Could you check a few things on this model? Use its own coordinates, in mm. Coordinates: 2 decimals unless noted, no trailing zeros. Loops run counter-clockwise (first coordinate to the right, second up) from the corner with the lowest first, then second, coordinate; pieces in that order, holes last. Notation, with made-up numbers: (60, 53) - (64, 53) arc R13 ccw to (64, 62) - close; hole circle Ø3 at (79, -2). An arc over 180 degrees is marked (long way). One line per item, written item: value. Start each with the question number.
(1) If we section it at A-A on z = -7.5: Count the separate pieces of the cut face and the enclosed holes in it, then the cut area to 3 significant figures.
(2) If we section it at B-B on x = 55.5: Write out the boundary of the cut face in (y, z), then the cut area to 3 significant figures.
(3) If I drill on line 1 along Z through (x, y) = (117.5, -1); line 2 along Z through (x, y) = (74, 1.05), over which ranges is the centre line in solid material (lowest first)? Write a range as from..to.
(4) I'm going to push a flat-ended pin straight in: P1, Ø1.5, axis at x = 102.5, y = 0.5, coming from the +Z side. Where does the tip first touch, or does it pass through?
```python
from build123d import *

# Parameters (mm, degrees)
F1_W          = 145.2
F1_H          = 32
F2_DEPTH      = 2
F3_DEPTH      = 2.001
F3_DEPTH_BACK = 2.001
F4_R          = 1


with BuildPart() as f2:
    # F1 (on Front) → F2 (new body, symmetric)
    with BuildSketch(Plane.XZ):
        with Locations((67.15, -2.5)):
            Rectangle(F1_W, F1_H)
    extrude(amount=F2_DEPTH, both=True)

    # F0 (on Front) → F3 (cut, two sides)
    with BuildSketch(Plane.XZ) as f3_sk:
        with BuildLine():
            Line((2.45, -12.5), (2.45, 13.5))
            Line((2.45, 13.5), (-2.45, 13.5))
            Line((-2.45, 13.5), (-2.45, -12.5))
            ThreePointArc((-2.45, -12.5), (-2.1571067812, -13.2071067812), (-1.45, -13.5))
            Line((-1.45, -13.5), (1.45, -13.5))
            ThreePointArc((1.45, -13.5), (2.1571067812, -13.2071067812), (2.45, -12.5))
        make_face()
        with BuildLine():
            Line((10.35, 13.5), (5.45, 13.5))
            Line((5.45, 13.5), (5.45, -12.5))
            ThreePointArc((5.45, -12.5), (5.7428932188, -13.2071067812), (6.45, -13.5))
            Line((6.45, -13.5), (9.35, -13.5))
            ThreePointArc((9.35, -13.5), (10.0571067812, -13.2071067812), (10.35, -12.5))
            Line((10.35, -12.5), (10.35, 13.5))
        make_face()
        with BuildLine():
            Line((18.25, 13.5), (13.35, 13.5))
            Line((13.35, 13.5), (13.35, -12.5))
            ThreePointArc((13.35, -12.5), (13.6428932188, -13.2071067812), (14.35, -13.5))
            Line((14.35, -13.5), (17.25, -13.5))
            ThreePointArc((17.25, -13.5), (17.9571067812, -13.2071067812), (18.25, -12.5))
            Line((18.25, -12.5), (18.25, 13.5))
        make_face()
        with BuildLine():
            Line((26.15, 13.5), (21.25, 13.5))
            Line((21.25, 13.5), (21.25, -12.5))
            ThreePointArc((21.25, -12.5), (21.5428932188, -13.2071067812), (22.25, -13.5))
            Line((22.25, -13.5), (25.15, -13.5))
            ThreePointArc((25.15, -13.5), (25.8571067812, -13.2071067812), (26.15, -12.5))
            Line((26.15, -12.5), (26.15, 13.5))
        make_face()
        with BuildLine():
            Line((34.05, 13.5), (29.15, 13.5))
            Line((29.15, 13.5), (29.15, -12.5))
            ThreePointArc((29.15, -12.5), (29.4428932188, -13.2071067812), (30.15, -13.5))
            Line((30.15, -13.5), (33.05, -13.5))
            ThreePointArc((33.05, -13.5), (33.7571067812, -13.2071067812), (34.05, -12.5))
            Line((34.05, -12.5), (34.05, 13.5))
        make_face()
        with BuildLine():
            Line((41.95, 13.5), (37.05, 13.5))
            Line((37.05, 13.5), (37.05, -12.5))
            ThreePointArc((37.05, -12.5), (37.3428932188, -13.2071067812), (38.05, -13.5))
            Line((38.05, -13.5), (40.95, -13.5))
            ThreePointArc((40.95, -13.5), (41.6571067812, -13.2071067812), (41.95, -12.5))
            Line((41.95, -12.5), (41.95, 13.5))
        make_face()
        with BuildLine():
            Line((49.85, 13.5), (44.95, 13.5))
            Line((44.95, 13.5), (44.95, -12.5))
            ThreePointArc((44.95, -12.5), (45.2428932188, -13.2071067812), (45.95, -13.5))
            Line((45.95, -13.5), (48.85, -13.5))
            ThreePointArc((48.85, -13.5), (49.5571067812, -13.2071067812), (49.85, -12.5))
            Line((49.85, -12.5), (49.85, 13.5))
        make_face()
        with BuildLine():
            Line((57.75, 13.5), (52.85, 13.5))
            Line((52.85, 13.5), (52.85, -12.5))
            ThreePointArc((52.85, -12.5), (53.1428932188, -13.2071067812), (53.85, -13.5))
            Line((53.85, -13.5), (56.75, -13.5))
            ThreePointArc((56.75, -13.5), (57.4571067812, -13.2071067812), (57.75, -12.5))
            Line((57.75, -12.5), (57.75, 13.5))
        make_face()
        with BuildLine():
            Line((65.65, 13.5), (60.75, 13.5))
            Line((60.75, 13.5), (60.75, -12.5))
            ThreePointArc((60.75, -12.5), (61.0428932188, -13.2071067812), (61.75, -13.5))
            Line((61.75, -13.5), (64.65, -13.5))
            ThreePointArc((64.65, -13.5), (65.3571067812, -13.2071067812), (65.65, -12.5))
            Line((65.65, -12.5), (65.65, 13.5))
        make_face()
        with BuildLine():
            Line((73.55, 13.5), (68.65, 13.5))
            Line((68.65, 13.5), (68.65, -12.5))
            ThreePointArc((68.65, -12.5), (68.9428932188, -13.2071067812), (69.65, -13.5))
            Line((69.65, -13.5), (72.55, -13.5))
            ThreePointArc((72.55, -13.5), (73.2571067812, -13.2071067812), (73.55, -12.5))
            Line((73.55, -12.5), (73.55, 13.5))
        make_face()
        with BuildLine():
            Line((81.45, 13.5), (76.55, 13.5))
            Line((76.55, 13.5), (76.55, -12.5))
            ThreePointArc((76.55, -12.5), (76.8428932188, -13.2071067812), (77.55, -13.5))
            Line((77.55, -13.5), (80.45, -13.5))
            ThreePointArc((80.45, -13.5), (81.1571067812, -13.2071067812), (81.45, -12.5))
            Line((81.45, -12.5), (81.45, 13.5))
        make_face()
        with BuildLine():
            Line((89.35, 13.5), (84.45, 13.5))
            Line((84.45, 13.5), (84.45, -12.5))
            ThreePointArc((84.45, -12.5), (84.7428932188, -13.2071067812), (85.45, -13.5))
            Line((85.45, -13.5), (88.35, -13.5))
            ThreePointArc((88.35, -13.5), (89.0571067812, -13.2071067812), (89.35, -12.5))
            Line((89.35, -12.5), (89.35, 13.5))
        make_face()
        with BuildLine():
            Line((97.25, 13.5), (92.35, 13.5))
            Line((92.35, 13.5), (92.35, -12.5))
            ThreePointArc((92.35, -12.5), (92.6428932188, -13.2071067812), (93.35, -13.5))
            Line((93.35, -13.5), (96.25, -13.5))
            ThreePointArc((96.25, -13.5), (96.9571067812, -13.2071067812), (97.25, -12.5))
            Line((97.25, -12.5), (97.25, 13.5))
        make_face()
        with BuildLine():
            Line((105.15, 13.5), (100.25, 13.5))
            Line((100.25, 13.5), (100.25, -12.5))
            ThreePointArc((100.25, -12.5), (100.5428932188, -13.2071067812), (101.25, -13.5))
            Line((101.25, -13.5), (104.15, -13.5))
            ThreePointArc((104.15, -13.5), (104.8571067812, -13.2071067812), (105.15, -12.5))
            Line((105.15, -12.5), (105.15, 13.5))
        make_face()
        with BuildLine():
            Line((113.05, 13.5), (108.15, 13.5))
            Line((108.15, 13.5), (108.15, -12.5))
            ThreePointArc((108.15, -12.5), (108.4428932188, -13.2071067812), (109.15, -13.5))
            Line((109.15, -13.5), (112.05, -13.5))
            ThreePointArc((112.05, -13.5), (112.7571067812, -13.2071067812), (113.05, -12.5))
            Line((113.05, -12.5), (113.05, 13.5))
        make_face()
        with BuildLine():
            Line((120.95, 13.5), (116.05, 13.5))
            Line((116.05, 13.5), (116.05, -12.5))
            ThreePointArc((116.05, -12.5), (116.3428932188, -13.2071067812), (117.05, -13.5))
            Line((117.05, -13.5), (119.95, -13.5))
            ThreePointArc((119.95, -13.5), (120.6571067812, -13.2071067812), (120.95, -12.5))
            Line((120.95, -12.5), (120.95, 13.5))
        make_face()
        with BuildLine():
            Line((128.85, 13.5), (123.95, 13.5))
            Line((123.95, 13.5), (123.95, -12.5))
            ThreePointArc((123.95, -12.5), (124.2428932188, -13.2071067812), (124.95, -13.5))
            Line((124.95, -13.5), (127.85, -13.5))
            ThreePointArc((127.85, -13.5), (128.5571067812, -13.2071067812), (128.85, -12.5))
            Line((128.85, -12.5), (128.85, 13.5))
        make_face()
        with BuildLine():
            Line((136.75, 13.5), (131.85, 13.5))
            Line((131.85, 13.5), (131.85, -12.5))
            ThreePointArc((131.85, -12.5), (132.1428932188, -13.2071067812), (132.85, -13.5))
            Line((132.85, -13.5), (135.75, -13.5))
            ThreePointArc((135.75, -13.5), (136.4571067812, -13.2071067812), (136.75, -12.5))
            Line((136.75, -12.5), (136.75, 13.5))
        make_face()
    extrude(amount=-F3_DEPTH, mode=Mode.SUBTRACT)
    extrude(f3_sk.sketch, amount=F3_DEPTH_BACK, mode=Mode.SUBTRACT)

    # F4
    f4_edges = [f2.edges().sort_by_distance(p)[0] for p in [
        (-5.45, 0, 13.5),
        (139.75, 0, 13.5),
        (139.75, 0, -18.5),
        (-5.45, 0, -18.5),
        (-2.45, 0, 13.5),
        (5.45, 0, 13.5),
        (13.35, 0, 13.5),
        (2.45, 0, 13.5),
        (18.25, 0, 13.5),
        (26.15, 0, 13.5),
        (10.35, 0, 13.5),
        (21.25, 0, 13.5),
        (29.15, 0, 13.5),
        (34.05, 0, 13.5),
        (37.05, 0, 13.5),
        (41.95, 0, 13.5),
        (44.95, 0, 13.5),
        (49.85, 0, 13.5),
        (52.85, 0, 13.5),
        (60.75, 0, 13.5),
        (57.75, 0, 13.5),
        (65.65, 0, 13.5),
        (68.65, 0, 13.5),
        (73.55, 0, 13.5),
        (76.55, 0, 13.5),
        (81.45, 0, 13.5),
        (84.45, 0, 13.5),
        (89.35, 0, 13.5),
        (92.35, 0, 13.5),
        (97.25, 0, 13.5),
        (100.25, 0, 13.5),
        (105.15, 0, 13.5),
        (108.15, 0, 13.5),
        (113.05, 0, 13.5),
        (116.05, 0, 13.5),
        (120.95, 0, 13.5),
        (123.95, 0, 13.5),
        (128.85, 0, 13.5),
        (131.85, 0, 13.5),
        (136.75, 0, 13.5),
    ]]
    fillet(f4_edges, radius=F4_R)


solid = f2.part
```
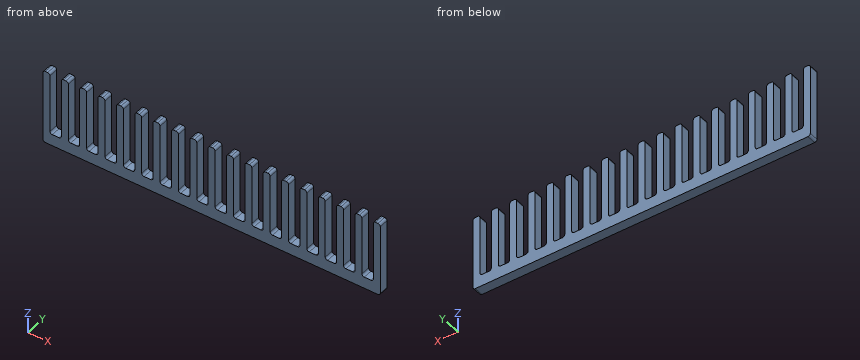
Values:
1. separate pieces: 19
1. enclosed holes: 0
1. area: 228 mm2
2. outline: (-2, -18.5) - (2, -18.5) - (2, -13.5) - (-2, -13.5) - close
2. area: 20.0 mm2
3. line 1: z = -18.5..-13.5
3. line 2: z = -18.5..13.34
4. P1: stops at z = -13.5
